```python
from build123d import *

# Parameters (mm, degrees)
SKETCH1_R           = 4.1
SKETCH1_R_2         = 2.05
BOSS_EXTRUDE1_DEPTH = 2
CUT_EXTRUDE1_DEPTH  = 95.490740287
FILLET1_DEPTH       = 2
FILLET2_R           = 10


with BuildPart() as part:
    # Sketch1 → Boss-Extrude1 (new body)
    with BuildSketch(Plane(origin=(0, 0, 0), x_dir=(1, 0, 0), z_dir=(0, 1, 0))):
        with BuildLine():
            Line((35, -10), (35, -23.5))
            Line((35, -23.5), (83, -23.5))
            ThreePointArc((83, -23.5), (91.5, -15), (83, -6.5))
            Line((83, -6.5), (48, -6.5))
            ThreePointArc((48, -6.5), (41.5, 0), (48, 6.5))
            Line((48, 6.5), (83, 6.5))
            ThreePointArc((83, 6.5), (91.5, 15), (83, 23.5))
            Line((83, 23.5), (35, 23.5))
            Line((35, 23.5), (35, 10))
            Line((35, 10), (0, 10))
            ThreePointArc((0, 10), (-10, 0), (0, -10))
            Line((0, -10), (35, -10))
        make_face()
        with Locations(Location((0, 0, 0), (0, 0, 270))):
            Circle(SKETCH1_R, mode=Mode.SUBTRACT)
        with Locations(Location((53, 15, 0), (0, 0, 270))):
            Circle(SKETCH1_R_2, mode=Mode.SUBTRACT)
        with Locations(Location((83, 15, 0), (0, 0, 270))):
            Circle(SKETCH1_R_2, mode=Mode.SUBTRACT)
        with Locations(Location((53, -15, 0), (0, 0, 270))):
            Circle(SKETCH1_R_2, mode=Mode.SUBTRACT)
        with Locations(Location((83, -15, 0), (0, 0, 270))):
            Circle(SKETCH1_R_2, mode=Mode.SUBTRACT)
    extrude(amount=BOSS_EXTRUDE1_DEPTH)

    # Sketch2 → Cut-Extrude1 (cut, through all)
    with BuildSketch(Plane(origin=(0, 2, 0), x_dir=(1, 0, 0), z_dir=(0, 1, 0))):
        with BuildLine():
            Line((-1.840672032, 8.554205192), (-1.4, 6.909594778))
            ThreePointArc((-1.4, 6.909594778), (0, 7.05), (1.4, 6.909594778))
            Line((1.4, 6.909594778), (1.840672032, 8.554205192))
            ThreePointArc((1.840672032, 8.554205192), (0, 8.75), (-1.840672032, 8.554205192))
        make_face()
    extrude(amount=-CUT_EXTRUDE1_DEPTH, mode=Mode.SUBTRACT)

    # Fillet1: read off the stored shape, not the designer's step
    # Fillet1 outline → Fillet1 (add)
    with BuildSketch(Plane(origin=(0, 0, 0), x_dir=(1, 0, 0), z_dir=(0, 1, 0))):
        with BuildLine():
            ThreePointArc((0, -10), (-0.41957616, -9.991193915), (-0.838413356, -9.964791169))
            ThreePointArc((-0.838413356, -9.964791169), (18.024740767, -14.233019392), (35, -23.5))
            Line((35, -23.5), (35, -10))
            Line((35, -10), (0, -10))
        make_face()
        with BuildLine():
            ThreePointArc((35, 23.5), (18.024740767, 14.233019392), (-0.838413356, 9.964791169))
            ThreePointArc((-0.838413356, 9.964791169), (-0.41957616, 9.991193915), (0, 10))
            Line((0, 10), (35, 10))
            Line((35, 10), (35, 23.5))
        make_face()
    extrude(amount=FILLET1_DEPTH)

    # Fillet2
    fillet2_edges = [part.edges().sort_by_distance(p)[0] for p in [
        (35, 1, -23.5),
        (35, 1, 23.5),
    ]]
    fillet(fillet2_edges, radius=FILLET2_R)


solid = part.part
```
Geometry check sheet. Reference: the model listing, model coordinates, mm. A direction names the side the tool comes from. Round coordinates to 2 decimals unless told otherwise and drop trailing zeros. Order: outer loops, then holes, each group sorted by start corner. A loop starts at its lowest first (then second) coordinate and runs counter-clockwise, first axis right, second up. Notation, with made-up numbers: (18.5, -4) - (64.5, -4) arc R21 ccw to (64.5, 21) - close; hole circle Ø5 at (-4, -24). An arc over 180 degrees is marked (long way). Use a Markdown table: item, result. Add a question column.
(1) Release check for a two-part mould opening along X. For faces 1 (the flat face through (65, 1, -6.5)), 2 (the cylindrical face through (55.033, 0.986, -15.267)), 3 (the cylindrical face through (35.208, 1.014, -23.047)) record: pulls with the +X half, pulls with the -X half, needs draft (parallel to the pull), parting line crosses it, or undercut.
(2) Material ranges on line 1 along Z through (x, y) = (79.5, 0.85); line 2 along X through (y, z) = (1.25, 15); line 3 along X through (y, z) = (1.7, -1), recorded low to high. Write a range as [from, to].
(3) Tool access check on faces 4 (the cylindrical face through (35.208, 1.014, 23.047)), 5 (the cylindrical face through (-0.02, 1.01, -7.05)), 6 (the flat face through (66, 1, 6.5)). Record the directions out of +Z, -Z, +X, -X, +Y, -Y that give a thin tool (end or side, any length) a straight path to the whole face; none if there is none.
(4) Sectioned sample at B-B, the plane x = 65. Enter the section's corners in (y, z).
(5) Sectioned sample at C-C, the plane y = 0.3. Enter the section's corners in (x, z), and give its area (3 significant figures).
(6) Sectioned sample at D-D, the plane z = -16. Enter the section's corners in (x, y) (3 decimals).
(7) Depth check by flat-ended pin: pin 1 (1 mm diameter, centred on y = 1.5, z = 1, fed in from +X). Enter the tip coordinate at first touch or a pass-through.
(8) Sectioned sample at A-A, the plane z = 0. Enter the section's corners in (x, y).
Answers below:
| question | item | result |
|---|---|---|
| 1 | face 1 | needs draft |
| 1 | face 2 | undercut |
| 1 | face 3 | pulls with the -X half |
| 2 | line 1 | [-23.5, -6.5], [6.5, 23.5] |
| 2 | line 2 | [19.97, 50.95], [55.05, 80.95], [85.05, 91.5] |
| 2 | line 3 | [-9.95, -3.98], [3.98, 41.58] |
| 3 | face 4 | +Z, -X, +Y, -Y |
| 3 | face 5 | +Y, -Y |
| 3 | face 6 | +X, +Y, -Y |
| 4 | outline | (0, -23.5) - (2, -23.5) - (2, -6.5) - (0, -6.5) - close; (0, 6.5) - (2, 6.5) - (2, 23.5) - (0, 23.5) - close |
| 5 | outline | (-0.84, -9.96) arc R70 cw to (32.57, -21.78) arc R10 ccw to (38.18, -23.5) - (83, -23.5) arc R8.5 ccw to (83, -6.5) - (48, -6.5) arc R6.5 cw to (48, 6.5) - (83, 6.5) arc R8.5 ccw to (83, 23.5) - (38.18, 23.5) arc R10 ccw to (32.57, 21.78) arc R70 cw to (-0.84, 9.96) arc R10 ccw to start; hole circle Ø8.2 at (0, 0); hole (-1.84, -8.55) arc R8.75 ccw to (1.84, -8.55) - (1.4, -6.91) arc R7.05 cw to (-1.4, -6.91) - close; hole circle Ø4.1 at (53, -15); hole circle Ø4.1 at (53, 15); hole circle Ø4.1 at (83, -15); hole circle Ø4.1 at (83, 15) |
| 5 | area | 3,050 mm² |
| 6 | outline | (22.275, 0) - (51.21, 0) - (51.21, 2) - (22.275, 2) - close; (54.79, 0) - (81.21, 0) - (81.21, 2) - (54.79, 2) - close; (84.79, 0) - (91.441, 0) - (91.441, 2) - (84.79, 2) - close |
| 7 | pin 1 | x = 41.68 |
| 8 | outline | (-10, 0) - (-4.1, 0) - (-4.1, 2) - (-10, 2) - close; (4.1, 0) - (41.5, 0) - (41.5, 2) - (4.1, 2) - close |
